Can you work these out from the model? Positions are in its coordinate system, mm. A direction names the side the tool comes from. Round coordinates to 2 decimals unless told otherwise and drop trailing zeros. Order: outer loops, then holes, each group sorted by start corner. A loop starts at its lowest first (then second) coordinate and runs counter-clockwise, first axis right, second up. Notation, with made-up numbers: (-25, 36.25) -> (-4, 36.25) arc R25 cw to (-4, 59.25) -> close; hole circle Ø5 at (89.25, 5.25). An arc over 180 degrees is marked (long way). Use a Markdown table: item, result. Add a question column.
Q1. I need wall thicknesses on line 1 along Z through (x, y) = (0, -0.15); line 2 along X through (y, z) = (-2.05, 0); line 3 along Y through (x, z) = (-4.5, -2.3). Which ranges of each line are inside material? Lowest first, please. Write a range as [from, to].
Q2. For faces 5 (the face through (-1.25, 2.5, 1.38)), 6 (the face through (2.4, -2, 0)), which set-ups out of +Z, -Z, +X, -X, +Y, -Y let a thin tool reach every point of the face, with its end or its side?
Q3. If we section it at A-A on y = 1.3: List the corners of the cut face in (x, z) for me, plus the area to 3 significant figures.
Q4. I'm going to push flat-ended pins straight in: pin 1 Ø3.5 at (x, z) = (4.5, 1) entering from -Y; pin 2 Ø3 at (y, z) = (-2.5, 0.5) entering from +X; pin 3 Ø1 at (y, z) = (-2, -0.5) entering from -X. Where does each tip first touch, or does it pass through?
Q5. If we section it at D-D on z = 1.9: List the corners of the cut face in (x, y) for me, plus the area to 3 significant figures.
Q6. We'd pull the mould along X, two halves only. Please class faces 1 (the face through (6, 1, 0)), 2 (the face through (-2.4, -2, 0)), 3 (the face through (-2, -3.5, 1)), 4 (the face through (-0.37, -0.46, 1.66)): +X half, -X half, draft (parallel to the pull), parting line (faces both ways), or undercut.
Q7. If we section it at B-B on x = 0: List the corners of the cut face in (y, z) for me, plus the area to 3 significant figures.
Q8. If we section it at C-C on z = 0: List the corners of the cut face in (x, y) for me.
```python
from build123d import *

# Parameters (mm, degrees)
BOSS_EXTRU_1_DEPTH      = 3
ESQUISSE2_R             = 1.7
ENL_V_MAT_EXTRU_1_DEPTH = 7
CONG_2_R                = 0.5


with BuildPart() as part:
    # Esquisse1 → Boss.-Extru.1 (new body, symmetric)
    with BuildSketch(Plane.XY):
        Polygon((-6, 0), (-2.4, 0), (-2.4, -3.5), (2.4, -3.5), (2.4, 0), (6, 0), (6, 2.5), (-6, 2.5), align=None)
    extrude(amount=BOSS_EXTRU_1_DEPTH, both=True)

    # Esquisse2 → Enlèv. mat.-Extru.1 (cut, through all)
    with BuildSketch(Plane(origin=(0, 2.5, 0), x_dir=(1, 0, 0), z_dir=(0, 1, 0))):
        Circle(ESQUISSE2_R)
    extrude(amount=-ENL_V_MAT_EXTRU_1_DEPTH, mode=Mode.SUBTRACT)

    # Congé2
    cong_2_edges = [part.edges().sort_by_distance(p)[0] for p in [
        (-6, 1.25, -3),
        (6, 1.25, -3),
        (-6, 1.25, 3),
        (-2.4, -1.75, 3),
        (2.4, -1.75, 3),
        (6, 1.25, 3),
        (2.4, -1.75, -3),
        (-2.4, -1.75, -3),
    ]]
    fillet(cong_2_edges, radius=CONG_2_R)


solid = part.part
```
Answer below:
| question | item | result |
|---|---|---|
| 1 | line 1 | [-3, -1.7], [1.7, 3] |
| 1 | line 2 | [-2.4, -1.7], [1.7, 2.4] |
| 1 | line 3 | [0, 2.5] |
| 2 | face 5 | +Z, -Z, +X, -X, +Y |
| 2 | face 6 | +Z, -Z, +X, -Y |
| 3 | outline | (-6, -2.5) arc R0.5 ccw to (-5.5, -3) -> (5.5, -3) arc R0.5 ccw to (6, -2.5) -> (6, 2.5) arc R0.5 ccw to (5.5, 3) -> (-5.5, 3) arc R0.5 ccw to (-6, 2.5) -> close; hole circle Ø3.4 at (0, 0) |
| 3 | area | 62.7 mm² |
| 4 | pin 1 | y = 0 |
| 4 | pin 2 | x = 2.4 |
| 4 | pin 3 | x = -2.4 |
| 5 | outline | (-6, 0) -> (-2.4, 0) -> (-2.4, -3.5) -> (2.4, -3.5) -> (2.4, 0) -> (6, 0) -> (6, 2.5) -> (-6, 2.5) -> close |
| 5 | area | 46.8 mm² |
| 6 | face 1 | +X half |
| 6 | face 2 | -X half |
| 6 | face 3 | draft |
| 6 | face 4 | undercut |
| 7 | outline | (-3.5, -3) -> (2.5, -3) -> (2.5, -1.7) -> (-3.5, -1.7) -> close; (-3.5, 1.7) -> (2.5, 1.7) -> (2.5, 3) -> (-3.5, 3) -> close |
| 7 | area | 15.6 mm² |
| 8 | outline | (-6, 0) -> (-2.4, 0) -> (-2.4, -3.5) -> (-1.7, -3.5) -> (-1.7, 2.5) -> (-6, 2.5) -> close; (1.7, -3.5) -> (2.4, -3.5) -> (2.4, 0) -> (6, 0) -> (6, 2.5) -> (1.7, 2.5) -> close |
